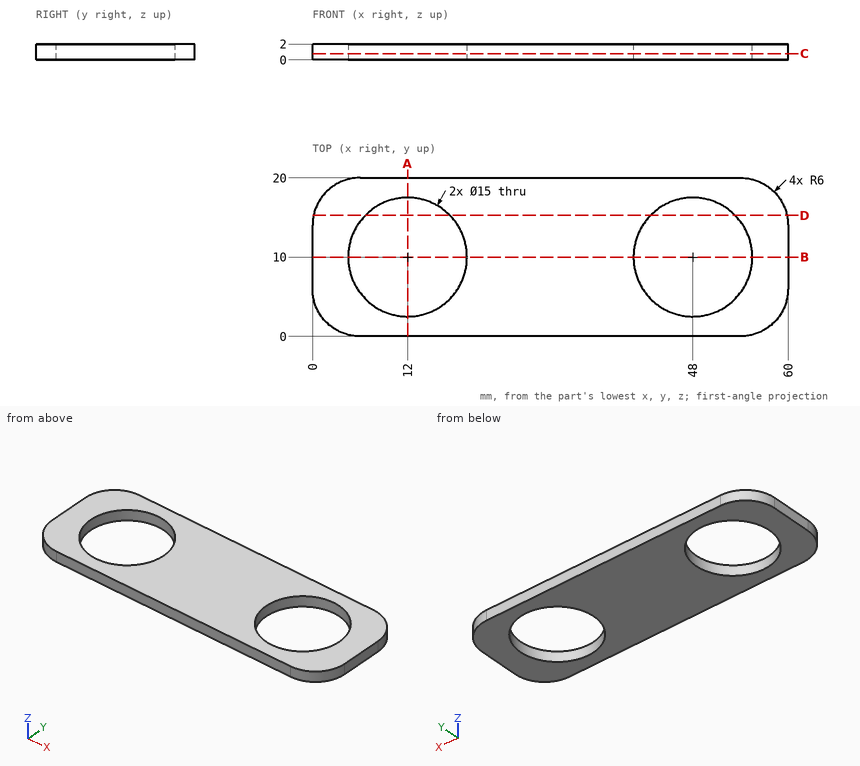
Answer from the drawing. Dimensions are ordinates in mm from the lowest x, y and z of the part. Coordinates: 2 decimals unless noted, no trailing zeros. Order: outer loops, then holes, each group sorted by start corner. A loop starts at its lowest first (then second) coordinate and runs counter-clockwise, first axis right, second up. Notation, with made-up numbers: (5.25, -27) - (37.25, -27) arc R19 cw to (37.25, -14) - close; hole circle Ø2 at (8.5, 12.25). An arc over 180 degrees is marked (long way). Put each result on its own line as item: value. Start each with the question number.
1) Find section D-D (y = 15.25). Give the vertices of the cut face in (x, z), plus the area to 3 significant figures.
2) Find section C-C (z = 0.8). Give the vertices of the cut face in (x, y), plus the area to 3 significant figures.
3) Find the intervals of material crossed by line 1 (Y direction, x = 12, z = 0.85); line 2 (X direction, y = 5.75, z = 0.8); line 3 (X direction, y = 13.75, z = 1.6), in increasing order. Write a range as from..to.
4) Find section B-B (y = 10). Give the vertices of the cut face in (x, z).
5) Find section A-A (x = 12). Give the vertices of the cut face in (y, z).
Results list:
1. outline: (0.13, 0) - (6.64, 0) - (6.64, 2) - (0.13, 2) - close; (17.36, 0) - (42.64, 0) - (42.64, 2) - (17.36, 2) - close; (53.36, 0) - (59.87, 0) - (59.87, 2) - (53.36, 2) - close
1. area: 76.6 mm^2
2. outline: (0, 6) arc R6 ccw to (6, 0) - (54, 0) arc R6 ccw to (60, 6) - (60, 14) arc R6 ccw to (54, 20) - (6, 20) arc R6 ccw to (0, 14) - close; hole circle Ø15 at (12, 10); hole circle Ø15 at (48, 10)
2. area: 816 mm^2
3. line 1: y = 0..2.5, 17.5..20
3. line 2: x = 0.01..5.82, 18.18..41.82, 54.18..59.99
3. line 3: x = 0..5.5, 18.5..41.5, 54.5..60
4. outline: (0, 0) - (4.5, 0) - (4.5, 2) - (0, 2) - close; (19.5, 0) - (40.5, 0) - (40.5, 2) - (19.5, 2) - close; (55.5, 0) - (60, 0) - (60, 2) - (55.5, 2) - close
5. outline: (0, 0) - (2.5, 0) - (2.5, 2) - (0, 2) - close; (17.5, 0) - (20, 0) - (20, 2) - (17.5, 2) - close
